from build123d import *

# Parameters (mm, degrees)
SKETCH1_W           = 150
SKETCH1_H           = 150
BOSS_EXTRUDE1_DEPTH = 15
CUT_EXTRUDE1_DEPTH  = 15
BOSS_EXTRUDE2_DEPTH = 25
CUT_EXTRUDE2_DEPTH  = 15
SKETCH5_R           = 2.5
CUT_EXTRUDE3_DEPTH  = 15
SKETCH7_R           = 2.5
CUT_EXTRUDE4_DEPTH  = 15
SKETCH8_R           = 3.8
CUT_EXTRUDE5_DEPTH  = 5
SKETCH10_R          = 2.5
CUT_EXTRUDE6_DEPTH  = 26
SKETCH11_R          = 3.8
CUT_EXTRUDE7_DEPTH  = 5
SKETCH12_R          = 2.5
CUT_EXTRUDE8_DEPTH  = 26
SKETCH13_R          = 3.8
CUT_EXTRUDE9_DEPTH  = 5
SKETCH14_R          = 2.5
CUT_EXTRUDE10_DEPTH = 26
SKETCH15_R          = 3.8
CUT_EXTRUDE11_DEPTH = 5
BOSS_EXTRUDE3_DEPTH = 15
BOSS_EXTRUDE4_DEPTH = 15
BOSS_EXTRUDE5_DEPTH = 15
BOSS_EXTRUDE6_DEPTH = 15
SKETCH20_W          = 7
SKETCH20_H          = 10
CUT_EXTRUDE12_DEPTH = 151
SKETCH21_W          = 7
SKETCH21_H          = 10
CUT_EXTRUDE13_DEPTH = 121


with BuildPart() as part:
    # Sketch1 → Boss-Extrude1 (new body)
    with BuildSketch(Plane.XY):
        Rectangle(SKETCH1_W, SKETCH1_H)
    extrude(amount=BOSS_EXTRUDE1_DEPTH)

    # Sketch2 → Cut-Extrude1 (cut)
    with BuildSketch(Plane.XY.offset(15)):
        Polygon((-41, 75), (-41, 60), (0, 20), (41, 60), (41, 75), align=None)
        Polygon((-20, 0), (-58, 45), (-75, 45), (-75, -45), (-58, -45), align=None)
        Polygon((58, 45), (20, 0), (58, -45), (75, -45), (75, 45), align=None)
        Polygon((41, -60), (0, -20), (-41, -60), (-41, -75), (41, -75), align=None)
    extrude(amount=-CUT_EXTRUDE1_DEPTH, mode=Mode.SUBTRACT)

    # Sketch3 → Boss-Extrude2 (add)
    with BuildSketch(Plane.XY.offset(15)):
        Polygon((-41, 45.069428085), (-58, 45.069428085), (-20, 0), (-58, -45), (-41, -45), (-41, -60), (0, -20), (41, -60), (41, -45), (58, -45), (20, 0), (58, 45), (41, 45), (41, 60), (0, 20), (-41, 60), align=None)
    extrude(amount=-BOSS_EXTRUDE2_DEPTH)

    # Sketch4 → Cut-Extrude2 (cut)
    with BuildSketch(Plane.XY.offset(15)):
        Polygon((-38, -42), (-38, -57.073170732), (0, -20), (38, -57.073170732), (38, -42), (55.466666667, -42), (20, 0), (55.466666667, 42), (37.925, 42), (37.925, 57), (0, 20), (-37.220661316, 56.312840308), (-37.426275475, 56.513439488), (-38, 57.073170732), (-38, 42), (-55.466666667, 42), (-20, 0), (-55.466666667, -42), align=None)
    extrude(amount=-CUT_EXTRUDE2_DEPTH, mode=Mode.SUBTRACT)

    # Sketch5 → Cut-Extrude3 (cut)
    with BuildSketch(Plane.XY):
        Circle(SKETCH5_R)
    extrude(amount=-CUT_EXTRUDE3_DEPTH, mode=Mode.SUBTRACT)

    # Sketch7 → Cut-Extrude4 (cut)
    with BuildSketch(Plane.XY.offset(15)):
        with Locations((70, -51)):
            Circle(SKETCH7_R)
        with Locations((46, -51)):
            Circle(SKETCH7_R)
        with Locations((46, -69)):
            Circle(SKETCH7_R)
        with Locations((70, -69)):
            Circle(SKETCH7_R)
    extrude(amount=-CUT_EXTRUDE4_DEPTH, mode=Mode.SUBTRACT)

    # Sketch8 → Cut-Extrude5 (cut)
    with BuildSketch(Plane.XY.offset(15)):
        with Locations((46, -51)):
            Circle(SKETCH8_R)
        with Locations((70, -51)):
            Circle(SKETCH8_R)
        with Locations((70, -69)):
            Circle(SKETCH8_R)
        with Locations((46, -69)):
            Circle(SKETCH8_R)
    extrude(amount=-CUT_EXTRUDE5_DEPTH, mode=Mode.SUBTRACT)

    # Sketch10 → Cut-Extrude6 (cut, through all)
    with BuildSketch(Plane.XY.offset(15)):
        with Locations((-46, -69)):
            Circle(SKETCH10_R)
        with Locations((-46, -51)):
            Circle(SKETCH10_R)
        with Locations((-70, -51)):
            Circle(SKETCH10_R)
        with Locations((-70, -69)):
            Circle(SKETCH10_R)
    extrude(amount=-CUT_EXTRUDE6_DEPTH, mode=Mode.SUBTRACT)

    # Sketch11 → Cut-Extrude7 (cut)
    with BuildSketch(Plane.XY.offset(15)):
        with Locations((-70, -51)):
            Circle(SKETCH11_R)
        with Locations((-46, -51)):
            Circle(SKETCH11_R)
        with Locations((-70, -69)):
            Circle(SKETCH11_R)
        with Locations((-46, -69)):
            Circle(SKETCH11_R)
    extrude(amount=-CUT_EXTRUDE7_DEPTH, mode=Mode.SUBTRACT)

    # Sketch12 → Cut-Extrude8 (cut, through all)
    with BuildSketch(Plane.XY.offset(15)):
        with Locations((46, 69)):
            Circle(SKETCH12_R)
        with Locations((70, 69)):
            Circle(SKETCH12_R)
        with Locations((70, 51)):
            Circle(SKETCH12_R)
        with Locations((46, 51)):
            Circle(SKETCH12_R)
    extrude(amount=-CUT_EXTRUDE8_DEPTH, mode=Mode.SUBTRACT)

    # Sketch13 → Cut-Extrude9 (cut)
    with BuildSketch(Plane.XY.offset(15)):
        with Locations((70, 69)):
            Circle(SKETCH13_R)
        with Locations((46, 69)):
            Circle(SKETCH13_R)
        with Locations((46, 51)):
            Circle(SKETCH13_R)
        with Locations((70, 51)):
            Circle(SKETCH13_R)
    extrude(amount=-CUT_EXTRUDE9_DEPTH, mode=Mode.SUBTRACT)

    # Sketch14 → Cut-Extrude10 (cut, through all)
    with BuildSketch(Plane.XY.offset(15)):
        with Locations((-70, 69)):
            Circle(SKETCH14_R)
        with Locations((-46, 69)):
            Circle(SKETCH14_R)
        with Locations((-46, 51)):
            Circle(SKETCH14_R)
        with Locations((-70, 51)):
            Circle(SKETCH14_R)
    extrude(amount=-CUT_EXTRUDE10_DEPTH, mode=Mode.SUBTRACT)

    # Sketch15 → Cut-Extrude11 (cut)
    with BuildSketch(Plane.XY.offset(15)):
        with Locations((-70, 69)):
            Circle(SKETCH15_R)
        with Locations((-46, 69)):
            Circle(SKETCH15_R)
        with Locations((-46, 51)):
            Circle(SKETCH15_R)
        with Locations((-70, 51)):
            Circle(SKETCH15_R)
    extrude(amount=-CUT_EXTRUDE11_DEPTH, mode=Mode.SUBTRACT)

    # Sketch16 → Boss-Extrude3 (add)
    with BuildSketch(Plane.XY):
        Polygon((-38, -57.073170732), (-23, -42.43902439), (-23, -27), (-42.8, -27), (-55.466666667, -42), (-38, -42), align=None)
    extrude(amount=BOSS_EXTRUDE3_DEPTH)

    # Sketch17 → Boss-Extrude4 (add)
    with BuildSketch(Plane.XY):
        Polygon((38, -57.073170732), (22.625, -42.073170732), (22.625, -27), (42.8, -27), (55.466666667, -42), (38, -42), align=None)
    extrude(amount=BOSS_EXTRUDE4_DEPTH)

    # Sketch18 → Boss-Extrude5 (add)
    with BuildSketch(Plane.XY):
        Polygon((37.925, 57), (22.925, 42.365853659), (22.925, 27), (42.8, 27), (55.466666667, 42), (37.925, 42), align=None)
    extrude(amount=BOSS_EXTRUDE5_DEPTH)

    # Sketch19 → Boss-Extrude6 (add)
    with BuildSketch(Plane.XY):
        Polygon((-38, 57.073170732), (-22.625, 42.073170732), (-22.625, 27), (-42.764877292, 27), (-55.466666667, 42), (-38, 42), align=None)
    extrude(amount=BOSS_EXTRUDE6_DEPTH)

    # Sketch20 → Cut-Extrude12 (cut, through all)
    with BuildSketch(Plane.XZ.offset(75)):
        with Locations((54.5, -5)):
            Rectangle(SKETCH20_W, SKETCH20_H)
    extrude(amount=-CUT_EXTRUDE12_DEPTH, mode=Mode.SUBTRACT)

    # Sketch21 → Cut-Extrude13 (cut, through all)
    with BuildSketch(Plane.XZ.offset(45)):
        with Locations((-54.5, -5)):
            Rectangle(SKETCH21_W, SKETCH21_H)
    extrude(amount=-CUT_EXTRUDE13_DEPTH, mode=Mode.SUBTRACT)


solid = part.part
Model file for the job. Use its own axes, mm. A direction names the side the tool comes from. Give positions to 0.01 mm unless a question says otherwise; leave off trailing zeros. Loops run counter-clockwise (first coordinate to the right, second up) from the corner with the lowest first, then second, coordinate; pieces in that order, holes last.
1) Saw through at A-A (z = 4.25). Count the separate pieces of the cut face and the enclosed holes in it, plus the area to 3 significant figures.
2) Saw through at C-C (z = -7.25). Write the cut outline in (x, y).
3) Wall check: line 1 (Y direction, x = -70, z = 7); line 2 (Y direction, x = 70, z = 12.3); line 3 (Y direction, x = 0, z = -3.5). Give the ranges that are in metal, low to high.
4) Flat gauge pins, fed straight in: pin 1 Ø3 at (x, z) = (-44.5, -6) entering from +Y; pin 2 Ø6 at (x, y) = (46, 69) entering from -Z; pin 3 Ø4 at (x, y) = (41.5, -47) entering from -Z; pin 4 Ø5 at (y, z) = (55.5, -6.5) entering from +X. Where does each tip first touch, or does it go through?
5) Tool access for faces 1 (the flat face through (-41, -67, 8)), 2 (the cylindrical face through (-66.49, -70.46, 12.54)), 3 (the flat face through (-23, -35, 7)), 4 (the flat face through (-22.625, 35, 7)): list every direction of +Z, -Z, +X, -X, +Y, -Y with a clear straight run to the whole face (end or side of a thin tool).
6) Saw through at B-B (y = -63). Write the cut outline in (x, z).
7) Pull direction X, two halves, no side cores. Call faces 5 (the flat face through (-41, 53, -5)), 6 (the flat face through (33, 27, 7)), 7 (the cylindrical face through (42.984, 66.688, 12.535)): +X half, -X half, draft (parallel to the pull), parting line (faces both ways), or undercut.
Answer block:
1. separate pieces: 4
1. enclosed holes: 16
1. area: 6,200 mm2
2. outline: (-51, -45) - (-41, -45) - (-41, -60) - (0, -20) - (41, -60) - (41, -45) - (51, -45) - (51, -36.71) - (20, 0) - (51, 36.71) - (51, 45) - (41, 45) - (41, 60) - (0, 20) - (-41, 60) - (-41, 45.07) - (-51, 45.07) - (-51, 36.77) - (-20, 0) - (-51, -36.71) - close; hole circle Ø5 at (0, 0)
3. line 1: y = -75 to -71.5, -66.5 to -53.5, -48.5 to -45, 45 to 48.5, 53.5 to 66.5, 71.5 to 75
3. line 2: y = -75 to -72.8, -65.2 to -54.8, -47.2 to -45, 45 to 47.2, 54.8 to 65.2, 72.8 to 75
3. line 3: y = -20 to -2.5, 2.5 to 20
4. pin 1: stops at y = 45.07
4. pin 2: stops at z = 0
4. pin 3: stops at z = -10
4. pin 4: stops at x = 41
5. face 1: +Z, -Z, -Y
5. face 2: +Z
5. face 3: +Z, -Y
5. face 4: +Z, +Y, -Y
6. outline: (-75, 0) - (-41, 0) - (-41, 15) - (-75, 15) - close; (41, 0) - (75, 0) - (75, 15) - (41, 15) - close
7. face 5: -X half
7. face 6: draft
7. face 7: undercut
